Geometry check sheet. Reference: the model listing, model coordinates, mm. A direction names the side the tool comes from. Give positions to 0.01 mm unless a question says otherwise; leave off trailing zeros. Loops run counter-clockwise (first coordinate to the right, second up) from the corner with the lowest first, then second, coordinate; pieces in that order, holes last.
1. Cross-section at A-A, the plane x = 44.1. Record the cut outline in (y, z), plus the area to 4 significant figures.
2. Release check for a two-part mould opening along Z. For faces 4 (the flat face through (66.64, 1.53, -26.11)), 5 (the cylindrical face through (-9.91, 1.6, -25.66)), 6 (the flat face through (-11.515, 3.236, -10.896)), 7 (the flat face through (27, 4, -2)) record: +Z half, -Z half, draft (parallel to the pull), parting line (faces both ways), or undercut.
3. Go/stop test with flat-tipped pins: pin 1 Ø1.5 at (x, z) = (63.5, -28) entering from -Y; pin 2 Ø5.5 at (x, z) = (-11.5, -27.5) entering from -Y; pin 3 Ø1 at (y, z) = (1, -48.5) entering from +X. Record where each tip stops, or that it passes through.
4. Material ranges on L1, parallel to X at y = 1.05, z = -41.25; L2, parallel to X at y = 1.95, z = 0; L3, parallel to Y at x = -7, z = -12.5, recorded low to high.
5. Cross-section at B-B, the plane z = -51.5. Record the cut outline in (x, y).
6. Cross-section at D-D, the plane z = 0. Record the cut outline in (x, y) (3 decimals).
7. Cross-section at C-C, the plane y = 0.8. State how many separate pieces and enclosed holes the cut face has, plus the area to 3 significant figures.
8. Tool access check on faces 1 (the cylindrical face through (61.605, 1.972, 3.288)), 2 (the cylindrical face through (63.28, 1.6, -13.42)), 3 (the cylindrical face through (54.73, 1.97, -4.75)). Record the directions out of +Z, -Z, +X, -X, +Y, -Y that give a thin tool (end or side, any length) a straight path to the whole face; none if there is none.
from build123d import *

# Parameters (mm, degrees)
BOSS_EXTRUDE1_DEPTH = 4
SKETCH5_R           = 2.5
CUT_EXTRUDE1_DEPTH  = 3.25
SKETCH6_W           = 30
SKETCH6_H           = 0.5
BOSS_EXTRUDE2_DEPTH = 6
BOSS_EXTRUDE3_DEPTH = 30
SKETCH8_W           = 30
SKETCH8_H           = 0.5
BOSS_EXTRUDE4_DEPTH = 6
BOSS_EXTRUDE5_DEPTH = 30


# Read off the part's stored shape, not the designer's step: M3x0.5 Tapped Hole1
with BuildPart() as part:
    # Sketch1 → Boss-Extrude1 (new body)
    with BuildSketch(Plane(origin=(0, 0, 0), x_dir=(1, 0, 0), z_dir=(0, 1, 0))):
        with BuildLine():
            Line((-26.885531635, 53.445375747), (-3.427655647, -2.16596819))
            ThreePointArc((-3.427655647, -2.16596819), (-2.322135184, -3.499790448), (-0.663506921, -4))
            Line((-0.663506921, -4), (59.665068599, -4))
            ThreePointArc((59.665068599, -4), (61.627788827, -3.268860795), (62.633827917, -1.431819537))
            Line((62.633827917, -1.431819537), (70.758345757, 54.424240617))
            ThreePointArc((70.758345757, 54.424240617), (67.375759383, 58.958345757), (62.841654243, 55.575759383))
            Line((62.841654243, 55.575759383), (55.713279127, 6.568180463))
            ThreePointArc((55.713279127, 6.568180463), (54.707240038, 4.731139205), (52.744519809, 4))
            Line((52.744519809, 4), (4.644548446, 4))
            ThreePointArc((4.644548446, 4), (2.985920183, 4.500209552), (1.88039972, 5.83403181))
            Line((1.88039972, 5.83403181), (-19.514468365, 56.554624253))
            ThreePointArc((-19.514468365, 56.554624253), (-24.754624253, 58.685531635), (-26.885531635, 53.445375747))
        make_face()
    extrude(amount=BOSS_EXTRUDE1_DEPTH)

    # M3x0.5 Tapped Hole1 outline → M3x0.5 Tapped Hole1 (revolve, cut)
    with BuildSketch(Plane(origin=(-23.2, 0, -55), x_dir=(1, 0, 0), z_dir=(0, 0, 1))):
        Polygon((0, 0), (1.25, 0), (1.25, 3.725), (1.525, 4), (0, 4), align=None)
    revolve(axis=Axis((-23.2, 0, -55), (0, 1, 0)), mode=Mode.SUBTRACT)

    # M3x0.5 Tapped Hole1 2 outline → M3x0.5 Tapped Hole1 2 (revolve, cut)
    with BuildSketch(Plane.XY):
        Polygon((0, 0), (1.25, 0), (1.25, 3.725), (1.525, 4), (0, 4), align=None)
    revolve(axis=Axis((0, 0, 0), (0, 1, 0)), mode=Mode.SUBTRACT)

    # M3x0.5 Tapped Hole1 3 outline → M3x0.5 Tapped Hole1 3 (revolve, cut)
    with BuildSketch(Plane(origin=(58.8, 0, 0), x_dir=(1, 0, 0), z_dir=(0, 0, 1))):
        Polygon((0, 0), (1.25, 0), (1.25, 3.725), (1.525, 4), (0, 4), align=None)
    revolve(axis=Axis((58.8, 0, 0), (0, 1, 0)), mode=Mode.SUBTRACT)

    # M3x0.5 Tapped Hole1 4 outline → M3x0.5 Tapped Hole1 4 (revolve, cut)
    with BuildSketch(Plane(origin=(66.8, 0, -55), x_dir=(1, 0, 0), z_dir=(0, 0, 1))):
        Polygon((0, 0), (1.25, 0), (1.25, 3.725), (1.525, 4), (0, 4), align=None)
    revolve(axis=Axis((66.8, 0, -55), (0, 1, 0)), mode=Mode.SUBTRACT)

    # Sketch5 → Cut-Extrude1 (cut)
    with BuildSketch(Plane.XZ):
        with Locations(Location((-17.4, -41.25, 0), (0, 0, 270))):
            Circle(SKETCH5_R)
        with Locations(Location((29.4, 0, 0), (0, 0, 270))):
            Circle(SKETCH5_R)
        with Locations(Location((60.8, -13.75, 0), (0, 0, 270))):
            Circle(SKETCH5_R)
        with Locations(Location((-5.8, -13.75, 0), (0, 0, 270))):
            Circle(SKETCH5_R)
        with Locations(Location((64.8, -41.25, 0), (0, 0, 270))):
            Circle(SKETCH5_R)
        with Locations(Location((-11.6, -27.5, 0), (0, 0, 270))):
            Circle(SKETCH5_R)
        with Locations(Location((14.7, 0, 0), (0, 0, 270))):
            Circle(SKETCH5_R)
        with Locations(Location((44.1, 0, 0), (0, 0, 270))):
            Circle(SKETCH5_R)
        with Locations(Location((62.8, -27.5, 0), (0, 0, 270))):
            Circle(SKETCH5_R)
    extrude(amount=-CUT_EXTRUDE1_DEPTH, mode=Mode.SUBTRACT)

    # Sketch6 → Boss-Extrude2 (add)
    with BuildSketch(Plane(origin=(-3.685531635, 0, 1.554624253), x_dir=(0.38865606330829405, 0, 0.921382908705007), z_dir=(-0.921382908705007, 0, 0.38865606330829405))):
        with Locations((-29.514686863, 3.75)):
            Rectangle(SKETCH6_W, SKETCH6_H)
    extrude(amount=BOSS_EXTRUDE2_DEPTH)

    # Sketch7 → Boss-Extrude3 (add)
    with BuildSketch(Plane(origin=(-5.641221056, 0, -13.373584401), x_dir=(0.9213829087050069, 0, -0.3886560633082941), z_dir=(0.3886560633082942, 0, 0.921382908705007))):
        Polygon((-4, 2), (-4, 3.5), (-10, 3.5), align=None)
    extrude(amount=-BOSS_EXTRUDE3_DEPTH)

    # Sketch8 → Boss-Extrude4 (add)
    with BuildSketch(Plane(origin=(61.540087421, 0, 8.951285443), x_dir=(0.14393984571411056, 0, -0.9895864392845114), z_dir=(0.9895864392845114, 0, 0.14393984571411056))):
        with Locations((35.820515092, 3.75)):
            Rectangle(SKETCH8_W, SKETCH8_H)
    extrude(amount=BOSS_EXTRUDE4_DEPTH)

    # Sketch9 → Boss-Extrude5 (add)
    with BuildSketch(Plane(origin=(2.99690173, 0, -20.603699394), x_dir=(0.9895864392845114, 0, 0.14393984571411056), z_dir=(-0.14393984571411056, 0, 0.9895864392845114))):
        Polygon((68.18768263, 3.5), (62.18768263, 3.5), (62.18768263, 2), align=None)
    extrude(amount=-BOSS_EXTRUDE5_DEPTH)


solid = part.part
Result:
1. outline: (0, -4) - (4, -4) - (4, 4) - (0, 4) - (0, 2.5) - (3.25, 2.5) - (3.25, -2.5) - (0, -2.5) - close
1. area: 15.75 mm2
2. face 4: undercut
2. face 5: undercut
2. face 6: +Z half
2. face 7: draft
3. pin 1: stops at y = 3.25
3. pin 2: stops at y = 0
3. pin 3: stops at x = 69.97
4. L1: x = -21.74 to -19.9, -14.9 to -13.06, 60.76 to 62.3, 67.3 to 68.84
4. L2: x = -4.34 to -1.25, 1.25 to 12.2, 17.2 to 26.9, 31.9 to 41.6, 46.6 to 57.55, 60.05 to 62.84
4. L3: y = 3.25 to 4
5. outline: (-26.06, 0) - (-17.38, 0) - (-17.38, 4) - (-26.06, 4) - close; (62.25, 0) - (70.33, 0) - (70.33, 4) - (62.25, 4) - close
6. outline: (-4.341, 0) - (-1.25, 0) - (-1.25, 3.725) - (-1.525, 4) - (-4.341, 4) - close; (1.25, 0) - (12.2, 0) - (12.2, 3.25) - (17.2, 3.25) - (17.2, 0) - (26.9, 0) - (26.9, 3.25) - (31.9, 3.25) - (31.9, 0) - (41.6, 0) - (41.6, 3.25) - (46.6, 3.25) - (46.6, 0) - (57.55, 0) - (57.55, 3.725) - (57.275, 4) - (1.525, 4) - (1.25, 3.725) - close; (60.05, 0) - (62.842, 0) - (62.842, 4) - (60.325, 4) - (60.05, 3.725) - close
7. separate pieces: 1
7. enclosed holes: 13
7. area: 1,250 mm2
8. face 1: +Z, +X, +Y, -Y
8. face 2: -Y
8. face 3: -Z, +Y, -Y
